Source: CAD feature listing. Evaluate the final solid. Frame: model axes, mm. Coordinates: 2 decimals unless noted, no trailing zeros. Order: outer loops, then holes, each group sorted by start corner. A loop starts at its lowest first (then second) coordinate and runs counter-clockwise, first axis right, second up.
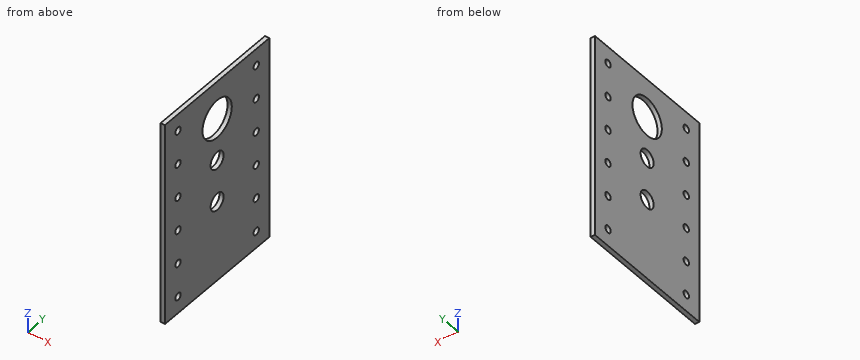
Autodesk Inventor part; units mm, degrees
ref_plane "YZ Plane" through (0, 0, 0) normal (1, 0, 0) x (0, 1, 0)
ref_plane "XZ Plane" through (0, 0, 0) normal (0, 1, 0) x (-1, 0, 0)
ref_plane "XY Plane" through (0, 0, 0) normal (0, 0, 1) x (1, 0, 0)
sketch "Sketch1" plane through (0, 0, 0) normal (1, 0, 0) x (0, 1, 0)
  line L0 (0, 0) -> (101.6, 0)
  line L1 (101.6, 0) -> (101.6, -152.4)
  line L2 (101.6, -152.4) -> (0, -152.4)
  line L3 (0, -152.4) -> (0, 0)
  circle A0 centre (50.8, -28.575) radius 14.2875
  circle A1 centre (50.8, -60.325) radius 6.35
  circle A2 centre (50.8, -92.075) radius 6.35
  circle A3 centre (50.8, -123.825) radius 14.2875
  line L4 (50.8, -28.575) -> (50.8, -123.825) construction
  circle A4 centre (88.9, -12.7) radius 2.6543
  circle A5 centre (88.9, -38.1) radius 2.6543
  circle A6 centre (88.9, -63.5) radius 2.6543
  circle A7 centre (88.9, -88.9) radius 2.6543
  circle A8 centre (88.9, -114.3) radius 2.6543
  circle A9 centre (88.9, -139.7) radius 2.6543
  circle A10 centre (12.7, -12.7) radius 2.6543
  circle A11 centre (12.7, -38.1) radius 2.6543
  circle A12 centre (12.7, -63.5) radius 2.6543
  circle A13 centre (12.7, -88.9) radius 2.6543
  circle A14 centre (12.7, -114.3) radius 2.6543
  circle A15 centre (12.7, -139.7) radius 2.6543
  point P0 (101.6, -76.2)
  point P1 (50.8, -76.2)
  point P2 (50.8, -152.4)
  dimension "d0" = 101.6
  dimension "d1" = 152.4
  dimension "d2" = 28.575
  dimension "d3" = 12.7
  dimension "d4" = 12.7
  dimension "d5" = 28.575
  dimension "d6" = 31.75
  dimension "d7" = 31.75
  dimension "d8" = 31.75
  dimension "d9" = 5.3086
  dimension "d10" = 12.7
  dimension "d11" = 12.7
  dimension "d14" = 25.4
  dimension "d17" = 76.2
extrude "Extrusion1" add sketch "Sketch1" along normal blind 3.175 contours L0 L1 L2 L3 | A3
equation "\"d7\" = d6"
equation "\"d8\" = d7"
properties part number "CH-1-02-RearGearboxHousingWheelSide"
1. Section query A-A on y = 88.9. Return loops of the section in (x, z) (3 decimals), plus the area to 3 significant figures.
Findings:
outline: (0, -152.4) - (3.175, -152.4) - (3.175, -142.354) - (0, -142.354) - close; (0, -137.046) - (3.175, -137.046) - (3.175, -116.954) - (0, -116.954) - close; (0, -111.646) - (3.175, -111.646) - (3.175, -91.554) - (0, -91.554) - close; (0, -86.246) - (3.175, -86.246) - (3.175, -66.154) - (0, -66.154) - close; (0, -60.846) - (3.175, -60.846) - (3.175, -40.754) - (0, -40.754) - close; (0, -35.446) - (3.175, -35.446) - (3.175, -15.354) - (0, -15.354) - close; (0, -10.046) - (3.175, -10.046) - (3.175, 0) - (0, 0) - close
area: 383 mm2
2. Ray query, line 1 (Z direction, x = 0.25, y = 46); line 2 (Y direction, x = 3.05, z = -39); line 3 (Y direction, x = 1.05, z = -92.5). Return the intervals inside material, ascending.
Findings:
line 1: z = -152.4 to -96.23, -87.92 to -64.48, -56.17 to -42.03, -15.12 to 0
line 2: y = 0 to 10.2, 15.2 to 41.03, 60.57 to 86.4, 91.4 to 101.6
line 3: y = 0 to 44.46, 57.14 to 101.6
3. Section query D-D on z = -31.5. Return loops of the section in (x, y) (3 decimals), plus the area to 3 significant figures.
Findings:
outline: (0, 0) - (3.175, 0) - (3.175, 36.815) - (0, 36.815) - close; (0, 64.785) - (3.175, 64.785) - (3.175, 101.6) - (0, 101.6) - close
area: 234 mm2
4. Pin query (flat end, axial travel): P1, Ø11.5, axis at y = 50.8, z = -60.325, coming from the -X side. Return the tip coordinate at first contact, or that it passes through.
Findings:
P1: passes through
5. Section query B-B on z = -12.7. Return loops of the section in (x, y) (3 decimals), plus the area to 3 significant figures.
Findings:
outline: (0, 0) - (3.175, 0) - (3.175, 10.046) - (0, 10.046) - close; (0, 15.354) - (3.175, 15.354) - (3.175, 86.246) - (0, 86.246) - close; (0, 91.554) - (3.175, 91.554) - (3.175, 101.6) - (0, 101.6) - close
area: 289 mm2
6. Section query C-C on y = 50.8. Return loops of the section in (x, z) (1 decimal).
Findings:
outline: (0, -152.4) - (3.2, -152.4) - (3.2, -98.4) - (0, -98.4) - close; (0, -85.7) - (3.2, -85.7) - (3.2, -66.7) - (0, -66.7) - close; (0, -54) - (3.2, -54) - (3.2, -42.9) - (0, -42.9) - close; (0, -14.3) - (3.2, -14.3) - (3.2, 0) - (0, 0) - close
